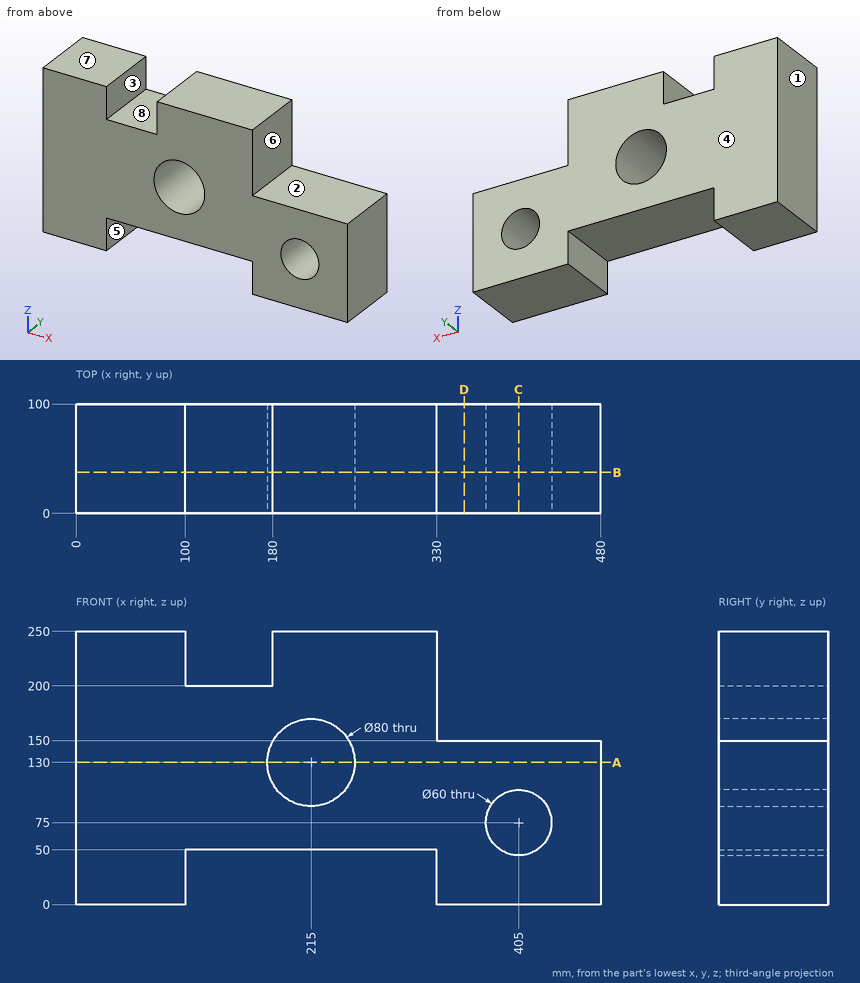
The figure shows three views and two pictorial views of one solid part (mm, origin at its lowest corner). Answer the questions. A direction names the side the tool comes from. Coordinates: 2 decimals unless noted, no trailing zeros. Loops run counter-clockwise (first coordinate to the right, second up) from the corner with the lowest first, then second, coordinate; pieces in that order, holes last. Notation, with made-up numbers: (88, 56) - (132, 56) arc R12 ccw to (132, 69) - close; hole circle Ø8 at (37, -37). An arc over 180 degrees is marked (long way). Write item = value, one per line.
1) Determine the mould class of the marked faces 6, 7 and 8 for opening direction X: pulls with the +X half, pulls with the -X half, needs draft (parallel to the pull), parting line crosses it, or undercut.
Responses:
face_6 = pulls with the +X half
face_7 = needs draft
face_8 = undercut
2) Find the intervals of material crossed by line 1 along Z through (x, y) = (215, 58); line 2 along Z through (x, y) = (405, 58); line 3 along X through (y, z) = (66, 75), in increasing order.
Responses:
line_1 = 50 to 90, 170 to 250
line_2 = 0 to 45, 105 to 150
line_3 = 0 to 375, 435 to 480
3) Section A-A (z = 130) is taken. Determine the outline of the cut face in (x, y).
Responses:
outline = (0, 0) - (175, 0) - (175, 100) - (0, 100) - close; (255, 0) - (480, 0) - (480, 100) - (255, 100) - close
4) Section B-B (y = 37.5) is taken. Determine the outline of the cut face in (x, z).
Responses:
outline = (0, 0) - (100, 0) - (100, 50) - (330, 50) - (330, 0) - (480, 0) - (480, 150) - (330, 150) - (330, 250) - (180, 250) - (180, 200) - (100, 200) - (100, 250) - (0, 250) - close; hole circle Ø80 at (215, 130); hole circle Ø60 at (405, 75)
5) Which of the six approach directions +Z, -Z, +X, -X, +Y, -Y give full straight-line access (tool end or side, diameter ignored) to the marked faces 1, 2, 3, 4 and 5?
Responses:
face_1 = +Z, -Z, -X, +Y, -Y
face_2 = +Z, +X, +Y, -Y
face_3 = +Z, +Y, -Y
face_4 = +Z, -Z, +X, -X, +Y
face_5 = -Z, +Y, -Y
6) Each of these flat-tipped pins is pushed along its axis until it touches: P1, Ø2, axis at x = 169, y = 82.5, coming from the -Z side; P2, Ø1, axis at x = 125.5, y = 70, coming from the +Z side. Where does it stop, or does it pass through?
Responses:
P1 = 50
P2 = 200
7) Section C-C (x = 405) is taken. Determine the outline of the cut face in (y, z).
Responses:
outline = (0, 0) - (100, 0) - (100, 45) - (0, 45) - close; (0, 105) - (100, 105) - (100, 150) - (0, 150) - close
8) Section D-D (x = 355) is taken. Determine the outline of the cut face in (y, z).
Responses:
outline = (0, 0) - (100, 0) - (100, 150) - (0, 150) - close
